Input: part model. Units: mm. Frame: model coordinates. Face numbers are marked on the shaded views. Give positions to 0.01 mm unless a question says otherwise; leave off trailing zeros. Return JSON: item names as keys, results as strings. Group by question number.
```python
from build123d import *

# Parameters (mm, degrees)
SKETCH_1_W      = 58
SKETCH_1_H      = 14
SKETCH_1_R      = 3.05
SKETCH_1_R_2    = 5.05
EXTRUDE_1_DEPTH = 4
FILLET_1_SIZE   = 2


with BuildPart() as part:
    # 草图1 → 凸台-拉伸1 (new body)
    with BuildSketch(Plane.XY):
        with Locations((23.125, 0)):
            Rectangle(SKETCH_1_W, SKETCH_1_H)
        Circle(SKETCH_1_R, mode=Mode.SUBTRACT)
        with Locations((46.25, 0)):
            Circle(SKETCH_1_R, mode=Mode.SUBTRACT)
        with Locations((23.125, 0)):
            Circle(SKETCH_1_R_2, mode=Mode.SUBTRACT)
    extrude(amount=EXTRUDE_1_DEPTH)

    # 圆角1
    # a fillet whose section is not a circle: 2 mm, written as the material it takes off along each edge
    with BuildSketch(Plane(origin=(0, 0, 4), x_dir=(1, 0, 0), z_dir=(0, -1, 0))) as fillet_1_piece_1:
        with BuildLine():
            Bezier((3.05, -FILLET_1_SIZE), (3.05, 0), (3.05 + FILLET_1_SIZE, 0), weights=[1, 0.014142136, 1])
            Line((3.05 + FILLET_1_SIZE, 0), (3.05, 0))
            Line((3.05, 0), (3.05, -FILLET_1_SIZE))
        make_face()
    revolve(axis=Axis((0, 0, 4), (0, 0, 1)), mode=Mode.SUBTRACT)
    with BuildSketch(Plane(origin=(46.25, 0, 4), x_dir=(1, 0, 0), z_dir=(0, -1, 0))) as fillet_1_piece_2:
        with BuildLine():
            Bezier((3.05, -FILLET_1_SIZE), (3.05, 0), (3.05 + FILLET_1_SIZE, 0), weights=[1, 0.014142136, 1])
            Line((3.05 + FILLET_1_SIZE, 0), (3.05, 0))
            Line((3.05, 0), (3.05, -FILLET_1_SIZE))
        make_face()
    revolve(axis=Axis((46.25, 0, 4), (0, 0, 1)), mode=Mode.SUBTRACT)


solid = part.part
```
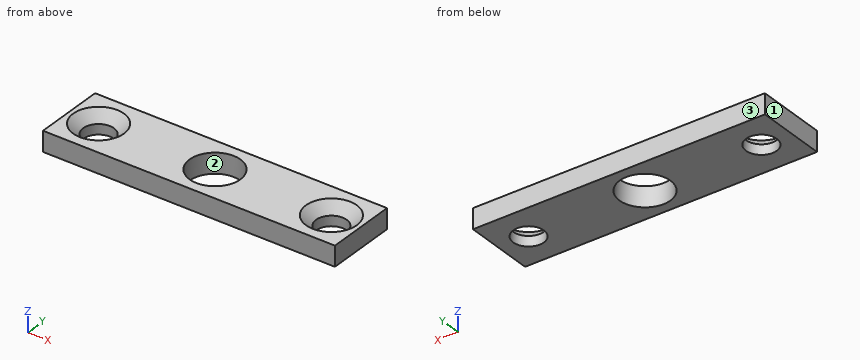
Item 1: Pull-direction query (Y, two-part tool) for the marked faces 1, 2 and 3; classes: pulls with the +Y half, pulls with the -Y half, needs draft (parallel to the pull), parting line crosses it, or undercut.
Item 2: Material intervals for line 1 (X direction, y = 0.25, z = 0.2) (3 decimals); line 2 (Y direction, x = 0, z = 1); line 3 (X direction, y = 2.25, z = 3.4) (3 decimals), sorted ascending. Write a range as from..to.
Item 3: Section A-A, the plane y = 0. Give the number of separate pieces and of enclosed holes in the cut face, then the cut area to 3 significant figures.
Item 4: First-contact query: pin 1 Ø5 at (x, y) = (0, 0) entering from -Z. Flat tip, straight axial feed; report the tip coordinate or a pass-through.
Answer below:
{
 "1": {"face 1": "needs draft", "face 2": "undercut", "face 3": "pulls with the +Y half"},
 "2": {"line 1": "-5.875..-3.04, 3.04..18.081, 28.169..43.21, 49.29..52.125", "line 2": "-7..-3.05, 3.05..7", "line 3": "-5.875..-3.809, 3.809..18.604, 27.646..42.441, 50.059..52.125"},
 "3": {"separate pieces": "4", "enclosed holes": "0", "area": "135 mm^2"},
 "4": {"pin 1": "through"}
}
